```python
from build123d import *

# Parameters (mm, degrees)
F0_R     = 10
F1_DEPTH = 20
F2_DEPTH = 30
F3_SIZE  = 2
F4_DEPTH = 40


with BuildPart() as f1:
    # F0 (on Front) → F1 (new body)
    with BuildSketch(Plane.XZ):
        with BuildLine():
            ThreePointArc((6.666667, 39.440532), (30.550505, 25.819889), (40, 0))
            ThreePointArc((40, 0), (30.550505, -25.819889), (6.666667, -39.440532))
            Line((6.666667, -39.440532), (123.333333, -19.720266))
            ThreePointArc((123.333333, -19.720266), (100, 0), (123.333333, 19.720266))
            Line((123.333333, 19.720266), (6.666667, 39.440532))
        make_face()
        with BuildLine():
            ThreePointArc((140, 0), (135.275252, 12.909944), (123.333333, 19.720266))
            ThreePointArc((123.333333, 19.720266), (100, 0), (123.333333, -19.720266))
            ThreePointArc((123.333333, -19.720266), (135.275252, -12.909944), (140, 0))
        make_face()
        with Locations((120, 0)):
            Circle(F0_R, mode=Mode.SUBTRACT)
        with BuildLine():
            ThreePointArc((6.666667, -39.440532), (30.550505, -25.819889), (40, 0))
            ThreePointArc((40, 0), (30.550505, 25.819889), (6.666667, 39.440532))
            ThreePointArc((6.666667, 39.440532), (-40, 0), (6.666667, -39.440532))
        make_face()
        Circle(F0_R, mode=Mode.SUBTRACT)
    extrude(amount=F1_DEPTH)

    # F0 (on Front) → F2 (join)
    with BuildSketch(Plane.XZ):
        with BuildLine():
            ThreePointArc((6.666667, -39.440532), (30.550505, -25.819889), (40, 0))
            ThreePointArc((40, 0), (30.550505, 25.819889), (6.666667, 39.440532))
            ThreePointArc((6.666667, 39.440532), (-40, 0), (6.666667, -39.440532))
        make_face()
        Circle(F0_R, mode=Mode.SUBTRACT)
    extrude(amount=-F2_DEPTH)

    # F3
    f3_edges = [f1.edges().sort_by_distance(p)[0] for p in [
        (-10, 30, 0),
        (-6.666667, 30, 39.440532),
        (110, 0, 0),
    ]]
    chamfer(f3_edges, length=F3_SIZE)

    # F0 (on Front) → F4 (join)
    with BuildSketch(Plane.XZ):
        with BuildLine():
            ThreePointArc((140, 0), (135.275252, 12.909944), (123.333333, 19.720266))
            ThreePointArc((123.333333, 19.720266), (100, 0), (123.333333, -19.720266))
            ThreePointArc((123.333333, -19.720266), (135.275252, -12.909944), (140, 0))
        make_face()
        with Locations((120, 0)):
            Circle(F0_R, mode=Mode.SUBTRACT)
    extrude(amount=-F4_DEPTH)


solid = f1.part
```
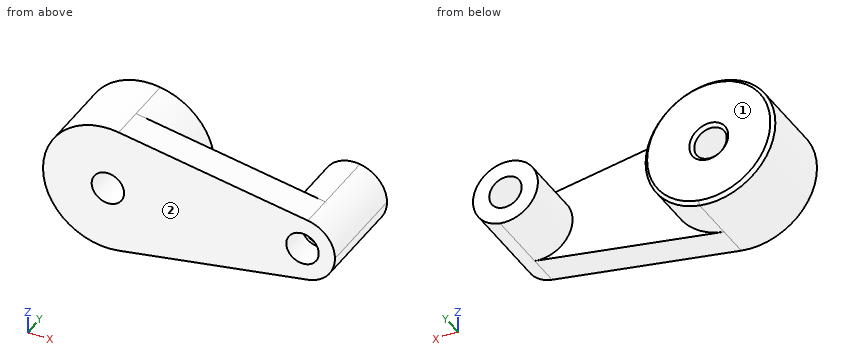
Input: part model. Units: mm. Frame: model coordinates. Face numbers are marked on the shaded views. A direction names the side the tool comes from. Give positions to 0.01 mm unless a question says otherwise; leave off trailing zeros. Order: outer loops, then holes, each group sorted by start corner. A loop starts at its lowest first (then second) coordinate and runs counter-clockwise, first axis right, second up. Notation, with made-up numbers: M -39,29.5 L -10,29.5 A19 ccw -10,50.5 Z; hole C -6.5,63.5 d11. An arc over 180 degrees is marked long. One line per question, with ' | ' between items. Start each with the question number.
1. Section query D-D (x = 69). Return the cut outline in (y, z), and give its area (3 significant figures).
2. First-contact query: pin 1 Ø3 at (y, z) = (12.5, -13) entering from -X; pin 2 Ø6 at (x, z) = (29, -29.5) entering from +Y; pin 3 Ø1 at (x, y) = (27.5, 20.5) entering from -Z. Flat tips, straight axial feed; report the tip coordinate or a pass-through.
3. Access query for the marked faces 1 and 2. Directions: +Z, -Z, +X, -X, +Y, -Y. A direction counts if a zero-diameter tool reaches every point of the face in a straight line with its end or side. Return the directions, or none.
4. Section query C-C (x = 104). Return the cut outline in (y, z).
5. Section query B-B (x = 0). Return the cut outline in (y, z).
6. Section query A-A (y = 10.5). Return the cut outline in (x, z), and give its area (3 significant figures).
7. Material intervals for probe 1 along Z at (x, y) = (0, -7); probe 2 along X at (y, z) = (15, -1); probe 3 along Z at (x, y) = (120, 15), sorted ascending. Write a range as [from, to].
Here are the results:
1) outline: M -20,-28.9 L 0,-28.9 L 0,28.9 L -20,28.9 Z | area: 1,160 mm²
2) pin 1: x = -38.31 | pin 2: y = 29.63 | pin 3: z = -29.51
3) face 1: +Z, -Z, -X, +Y | face 2: +Z, -Z, +X, -X, -Y
4) outline: M -20,-22.99 L 0,-22.99 L 0,-12 L 40,-12 L 40,12 L 0,12 L 0,22.99 L -20,22.99 Z
5) outline: M -20,-40 L 28,-40 L 30,-38 L 30,-12 L 28,-10 L -20,-10 Z; M -20,10 L 28,10 L 30,12 L 30,38 L 28,40 L -20,40 Z
6) outline: C 0,0 d80; M 123.33,-19.72 A20 ccw 140,0 A20 ccw 123.33,19.72 A20 ccw long Z; hole C 0,0 d20; hole C 120,0 d20 | area: 5,650 mm²
7) probe 1: [-40, -10], [10, 40] | probe 2: [-39.99, -9.95], [9.95, 39.99], [100.03, 110.05], [129.95, 139.97] | probe 3: [-20, -10], [10, 20]
